```python
from build123d import *

# Parameters (mm, degrees)
F0_R     = 38.1
F1_DEPTH = 12.7
F2_R     = 4
F3_DEPTH = 50


with BuildPart() as f1:
    # F0 (on Top) → F1 (new body)
    with BuildSketch(Plane.XY):
        Circle(F0_R)
    extrude(amount=F1_DEPTH)

    # F2 (on Right) → F3 (cut, symmetric)
    with BuildSketch(Plane.YZ):
        with Locations((-32.5239, 6.35)):
            Circle(F2_R)
        with Locations((-19.8239, 6.35)):
            Circle(F2_R)
        with Locations((-7.1239, 6.35)):
            Circle(F2_R)
        with Locations((5.5761, 6.35)):
            Circle(F2_R)
        with Locations((18.2761, 6.35)):
            Circle(F2_R)
        with Locations((30.9761, 6.35)):
            Circle(F2_R)
    extrude(amount=F3_DEPTH, both=True, mode=Mode.SUBTRACT)


solid = f1.part
```
The model under review builds one solid part; all positions refer to its coordinate system, in mm. Give positions to 0.01 mm unless a question says otherwise; leave off trailing zeros. Write each loop counter-clockwise with the first axis right and the second up, starting at its lowest first coordinate (ties: lowest second). Pieces come first, ordered by that corner, then holes.
(1) Consider section B-B, the plane x = -21. Give the boundary of the cut face in (y, z).
(2) The part is to be moulded in two halves that separate along Y. For faces 1 (the flat face through (-1, 1, 12.7)), 2 (the cylindrical face through (0.38, 26.98, 6.53)), 3 (the cylindrical face through (-28.08, 25.75, 6.26)), say which applies: released by +Y, released by -Y, zero draft, split by the parting line, or undercut.
(3) For P1, Ø3, axis at x = -2.5, z = 2.5, coming from the -Y side; P2, Ø5, axis at y = -7.12, z = 6.35, coming from the +X side; P3, Ø3, axis at y = -26.5, z = 9.5, coming from the +X side; P4, Ø3, axis at x = 30, z = 9.5, coming from the +Y side, all flat-tipped, find the tip position at first contact; note any pin that passes through.
(4) To check wall thickness, follow L1, parallel to Y at x = -18.5, z = 6.35; L2, parallel to Z at x = 5, y = -19.5; L3, parallel to Y at x = 30, z = 3. State the ranges of each line that lie inside material, in increasing order.
(5) Consider section C-C, the plane z = 6.35. Give the boundary of the cut face in (x, y), and give its area (3 significant figures).
(6) Consider section A-A, the plane y = 8. Give the boundary of the cut face in (x, z), and give its area (3 significant figures).
(7) Consider section D-D, the plane x = 5. Give the boundary of the cut face in (y, z).
Returned:
1. outline: (-31.79, 0) - (31.79, 0) - (31.79, 2.43) arc R4 cw (long way) to (31.79, 10.27) - (31.79, 12.7) - (-31.79, 12.7) - (-31.79, 10.28) arc R4 cw to (-31.79, 2.42) - close; hole circle Ø8 at (-19.82, 6.35); hole circle Ø8 at (-7.12, 6.35); hole circle Ø8 at (5.58, 6.35); hole circle Ø8 at (18.28, 6.35)
2. face 1: zero draft
2. face 2: undercut
2. face 3: split by the parting line
3. P1: stops at y = -38.09
3. P2: passes through
3. P3: stops at x = 28.75
3. P4: stops at y = 25.29
4. L1: y = -28.52 to -23.82, -15.82 to -11.12, -3.12 to 1.58, 9.58 to 14.28, 22.28 to 26.98
4. L2: z = 0 to 2.36, 10.34 to 12.7
4. L3: y = -23.49 to -22.01, -17.64 to -9.31, -4.94 to 3.39, 7.76 to 16.09, 20.46 to 23.49
5. outline: (-38.07, 1.58) arc R38.1 ccw to (-37.97, -3.12) - (37.97, -3.12) arc R38.1 ccw to (38.07, 1.58) - close; (-36.88, 9.58) - (36.88, 9.58) arc R38.1 ccw to (35.32, 14.28) - (-35.32, 14.28) arc R38.1 ccw to start; (-36.44, -11.12) arc R38.1 ccw to (-34.66, -15.82) - (34.66, -15.82) arc R38.1 ccw to (36.44, -11.12) - close; (-30.91, 22.28) - (30.91, 22.28) arc R38.1 ccw to (26.91, 26.98) - (-26.91, 26.98) arc R38.1 ccw to start; (-29.73, -23.82) arc R38.1 ccw to (-25.26, -28.52) - (25.26, -28.52) arc R38.1 ccw to (29.73, -23.82) - close; (-15.11, 34.98) - (15.11, 34.98) arc R38.1 ccw to start; (-10.85, -36.52) arc R38.1 ccw to (10.85, -36.52) - close
5. area: 1,650 mm2
6. outline: (-37.25, 0) - (37.25, 0) - (37.25, 3.17) - (-37.25, 3.17) - close; (-37.25, 9.53) - (37.25, 9.53) - (37.25, 12.7) - (-37.25, 12.7) - close
6. area: 472 mm2
7. outline: (-37.77, 0) - (37.77, 0) - (37.77, 12.7) - (-37.77, 12.7) - close; hole circle Ø8 at (-32.52, 6.35); hole circle Ø8 at (-19.82, 6.35); hole circle Ø8 at (-7.12, 6.35); hole circle Ø8 at (5.58, 6.35); hole circle Ø8 at (18.28, 6.35); hole circle Ø8 at (30.98, 6.35)
